The model under review builds one solid part; all positions refer to its coordinate system, in mm. Coordinates: 2 decimals unless noted, no trailing zeros. Order: outer loops, then holes, each group sorted by start corner. A loop starts at its lowest first (then second) coordinate and runs counter-clockwise, first axis right, second up. Notation, with made-up numbers: (43.25, 85) -> (89.25, 85) arc R25 cw to (89.25, 111) -> close; hole circle Ø8 at (6.5, -21). An arc over 180 degrees is marked (long way). Use one line per item in the form item = value.
from build123d import *

# Parameters (mm, degrees)
F0_W     = 19.05
F0_H     = 19.05
F1_DEPTH = 9.525
F2_SIZE  = 5.08


with BuildPart() as f1:
    # F0 (on Front) → F1 (new body, symmetric)
    with BuildSketch(Plane.XZ):
        Rectangle(F0_W, F0_H)
    extrude(amount=F1_DEPTH, both=True)

    # F2
    f2_edges = [f1.edges().sort_by_distance(p)[0] for p in [
        (0, -9.525, 9.525),
    ]]
    chamfer(f2_edges, length=F2_SIZE)


solid = f1.part
Item 1: To check wall thickness, follow L1, parallel to Y at x = -5.5, z = 7 (3 decimals); L2, parallel to Y at x = -3.75, z = 6.25 (3 decimals); L3, parallel to Z at x = -7.5, y = -6.5 (3 decimals). State the ranges of each line that lie inside material, in increasing order. Write a range as from..to.
Results found:
L1 = -6.97..9.525
L2 = -7.72..9.525
L3 = -9.525..7.47
Item 2: We need section C-C (x = 7.25). Write out the cut boundary in (y, z) (3 decimals), plus the area to 3 significant figures.
Results found:
outline = (-9.525, -9.525) -> (9.525, -9.525) -> (9.525, 9.525) -> (-4.445, 9.525) -> (-9.525, 4.445) -> close
area = 350 mm²
Item 3: We need section B-B (z = 5.75). Write out the cut boundary in (x, y) (3 decimals), plus the area to 3 significant figures.
Results found:
outline = (-9.525, -8.22) -> (9.525, -8.22) -> (9.525, 9.525) -> (-9.525, 9.525) -> close
area = 338 mm²
Item 4: We need section A-A (y = -6.75). Write out the cut boundary in (x, z) (3 decimals), plus the area to 3 significant figures.
Results found:
outline = (-9.525, -9.525) -> (9.525, -9.525) -> (9.525, 7.22) -> (-9.525, 7.22) -> close
area = 319 mm²
